Answer from the drawing. Dimensions are ordinates in mm from the lowest x, y and z of the part. A direction names the side the tool comes from. Give positions to 0.01 mm unless a question says otherwise; leave off trailing zeros. Order: outer loops, then holes, each group sorted by start corner. A loop starts at its lowest first (then second) coordinate and runs counter-clockwise, first axis right, second up. Notation, with made-up numbers: (-28.75, 31) -> (19.25, 31) arc R31 cw to (19.25, 63) -> close; hole circle Ø10 at (86.25, 34.25). An arc over 180 degrees is marked (long way). Answer as a JSON object with one key per item and string values. Group by question number.
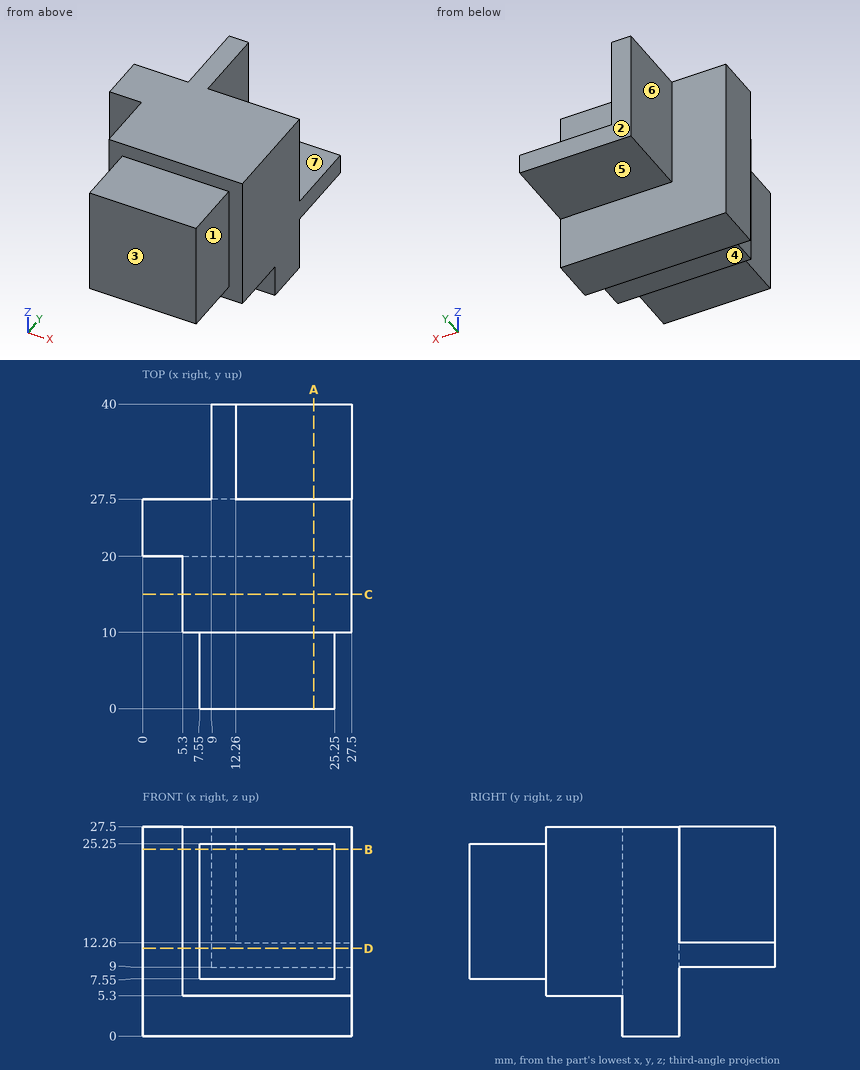
(1) Which of the six approach directions +Z, -Z, +X, -X, +Y, -Y give full straight-line access (tool end or side, diameter ignored) to the marked faces 4, 5, 6 and 7?
(2) Find the intervals of material crossed by line 1 along Z through (x, y) = (14.75, 2); line 2 along Y through (x, z) = (6.5, 3); line 3 along Y through (x, z) = (25.5, 7), in increasing order. Write a range as [from, to].
(3) A cutting plane is placed at A-A (x = 22.5). Determine the outline of the cut face in (y, z).
(4) A cutting plane is placed at D-D (z = 11.5). Determine the outline of the cut face in (x, y).
(5) A cutting plane is placed at C-C (y = 15). Determine the outline of the cut face in (x, z).
(6) A cutting plane is placed at B-B (z = 24.5). Determine the outline of the cut face in (x, y), and give its area (3 significant figures).
(7) For a pull along Y with two mould halves and no side action, classify the marked faces 1, 2 and 3 as +Y half, -Y half, draft (parallel to the pull), parting line (faces both ways), or undercut.
(8) Flat-ended cylindrical pins translate along their axes: pin 1 Ø1.5 at (y, z) = (35.5, 22.5) entering from +X; pin 2 Ø11 at (y, z) = (4, 19) entering from +X; pin 3 Ø3 at (x, z) = (17, 3) entering from -Y. Find the tip coordinate at first contact, or state that the pin passes through.
Check sheet entries:
{
 "1": {"face 4": "-Z, +X, -X, -Y", "face 5": "-Z, +X, -X, +Y", "face 6": "+Z, -Z, -X, +Y", "face 7": "+Z, +X, +Y"},
 "2": {"line 1": "z = [7.55, 25.25]", "line 2": "y = [20, 27.5]", "line 3": "y = [10, 27.5]"},
 "3": {"outline": "(0, 7.55) -> (10, 7.55) -> (10, 5.3) -> (20, 5.3) -> (20, 0) -> (27.5, 0) -> (27.5, 9) -> (40, 9) -> (40, 12.26) -> (27.5, 12.26) -> (27.5, 27.5) -> (10, 27.5) -> (10, 25.25) -> (0, 25.25) -> close"},
 "4": {"outline": "(0, 20) -> (5.3, 20) -> (5.3, 10) -> (7.55, 10) -> (7.55, 0) -> (25.25, 0) -> (25.25, 10) -> (27.5, 10) -> (27.5, 40) -> (9, 40) -> (9, 27.5) -> (0, 27.5) -> close"},
 "5": {"outline": "(5.3, 5.3) -> (27.5, 5.3) -> (27.5, 27.5) -> (5.3, 27.5) -> close"},
 "6": {"outline": "(0, 20) -> (5.3, 20) -> (5.3, 10) -> (7.55, 10) -> (7.55, 0) -> (25.25, 0) -> (25.25, 10) -> (27.5, 10) -> (27.5, 27.5) -> (12.26, 27.5) -> (12.26, 40) -> (9, 40) -> (9, 27.5) -> (0, 27.5) -> close", "area": "646 mm2"},
 "7": {"face 1": "draft", "face 2": "+Y half", "face 3": "-Y half"},
 "8": {"pin 1": "stops at x = 12.26", "pin 2": "stops at x = 25.25", "pin 3": "stops at y = 20"}
}
